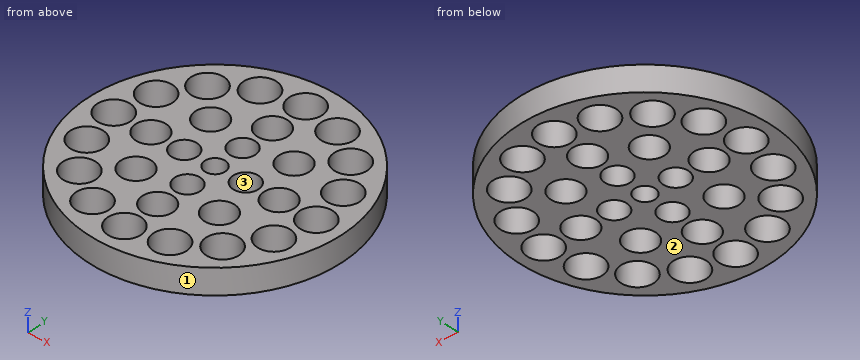
from build123d import *

# Parameters (mm, degrees)
F0_R     = 25
F0_R_2   = 3.25
F0_R_3   = 3
F0_R_4   = 2.5
F0_R_5   = 2
F1_DEPTH = 5


with BuildPart() as f1:
    # F0 (on Top) → F1 (new body)
    with BuildSketch(Plane.XY):
        Circle(F0_R)
        with Locations((-13.965359, -13.965359)):
            Circle(F0_R_2, mode=Mode.SUBTRACT)
        with Locations((-7.557998, -18.246621)):
            Circle(F0_R_2, mode=Mode.SUBTRACT)
        with Locations((-18.246621, -7.557998)):
            Circle(F0_R_2, mode=Mode.SUBTRACT)
        with Locations((-8.131728, -8.131728)):
            Circle(F0_R_3, mode=Mode.SUBTRACT)
        with Locations((0, -19.75)):
            Circle(F0_R_2, mode=Mode.SUBTRACT)
        with Locations((7.557998, -18.246621)):
            Circle(F0_R_2, mode=Mode.SUBTRACT)
        with Locations((13.965359, -13.965359)):
            Circle(F0_R_2, mode=Mode.SUBTRACT)
        with Locations((0, -12.5)):
            Circle(F0_R_3, mode=Mode.SUBTRACT)
        with Locations((8.131728, -8.131728)):
            Circle(F0_R_3, mode=Mode.SUBTRACT)
        with Locations((0, -6)):
            Circle(F0_R_4, mode=Mode.SUBTRACT)
        with Locations((18.246621, -7.557998)):
            Circle(F0_R_2, mode=Mode.SUBTRACT)
        with Locations((-19.75, 0)):
            Circle(F0_R_2, mode=Mode.SUBTRACT)
        with Locations((-18.246621, 7.557998)):
            Circle(F0_R_2, mode=Mode.SUBTRACT)
        with Locations((-12.5, 0)):
            Circle(F0_R_3, mode=Mode.SUBTRACT)
        with Locations((-6, 0)):
            Circle(F0_R_4, mode=Mode.SUBTRACT)
        with Locations((-8.131728, 8.131728)):
            Circle(F0_R_3, mode=Mode.SUBTRACT)
        with Locations((-13.965359, 13.965359)):
            Circle(F0_R_2, mode=Mode.SUBTRACT)
        with Locations((-7.557998, 18.246621)):
            Circle(F0_R_2, mode=Mode.SUBTRACT)
        Circle(F0_R_5, mode=Mode.SUBTRACT)
        with Locations((6, 0)):
            Circle(F0_R_4, mode=Mode.SUBTRACT)
        with Locations((0, 6)):
            Circle(F0_R_4, mode=Mode.SUBTRACT)
        with Locations((8.131728, 8.131728)):
            Circle(F0_R_3, mode=Mode.SUBTRACT)
        with Locations((12.5, 0)):
            Circle(F0_R_3, mode=Mode.SUBTRACT)
        with Locations((19.75, 0)):
            Circle(F0_R_2, mode=Mode.SUBTRACT)
        with Locations((18.246621, 7.557998)):
            Circle(F0_R_2, mode=Mode.SUBTRACT)
        with Locations((0, 12.5)):
            Circle(F0_R_3, mode=Mode.SUBTRACT)
        with Locations((7.557998, 18.246621)):
            Circle(F0_R_2, mode=Mode.SUBTRACT)
        with Locations((0, 19.75)):
            Circle(F0_R_2, mode=Mode.SUBTRACT)
        with Locations((13.965359, 13.965359)):
            Circle(F0_R_2, mode=Mode.SUBTRACT)
    extrude(amount=F1_DEPTH)


solid = f1.part
Read the model definition and answer for the solid it produces. Units are mm, in the model's axes. Face numbers are marked on the shaded views. Round coordinates to 2 decimals unless told otherwise and drop trailing zeros. Loops run counter-clockwise (first coordinate to the right, second up) from the corner with the lowest first, then second, coordinate; pieces in that order, holes last.
Q1. Section A-A on y = 0 is taken. Give the number of separate pieces and of enclosed holes in the cut face, and give its area (3 significant figures).
Q2. Consider probe 1 along Y at (x, z) = (6.5, 4.35); probe 2 along X at (y, z) = (13.5, 3.55); probe 3 along Y at (x, z) = (-5.5, 1). Determine where each line is inside the solid, lowest interval first.
Q3. Section B-B on x = 13.5 is taken. Write down the section's boundary in (y, z).
Q4. Each of these flat-tipped pins is pushed along its axis until it touches: pin 1 (3 mm diameter, centred on x = 4.5, z = 3, fed in from +Y); pin 2 (3 mm diameter, centred on x = 0, y = 0, fed in from -Z); pin 3 (1 mm diameter, centred on y = 15, z = 1.5, fed in from +X). Where does it stop, or does it pass through?
Q5. Determine the mould class of the marked faces 1, 2 and 3 for opening direction Y: released by +Y, released by -Y, zero draft, split by the parting line, or undercut.
Q6. Section C-C on y = 6 is taken. Write down the section's boundary in (x, z).
Output:
1. separate pieces: 8
1. enclosed holes: 0
1. area: 55.0 mm2
2. probe 1: y = -24.14 to -21.32, -15.17 to -10.65, -5.61 to -2.45, 2.45 to 5.61, 10.65 to 15.17, 21.32 to 24.14
2. probe 2: x = -21.04 to -17.18, -10.75 to -2.83, 2.83 to 10.75, 17.18 to 21.04
2. probe 3: y = -24.39 to -20.76, -15.73 to -9.57, -6.69 to -2.45, 2.45 to 6.69, 9.57 to 15.73, 20.76 to 24.39
3. outline: (-21.04, 0) - (-17.18, 0) - (-17.18, 5) - (-21.04, 5) - close; (-10.75, 0) - (-2.83, 0) - (-2.83, 5) - (-10.75, 5) - close; (2.83, 0) - (10.75, 0) - (10.75, 5) - (2.83, 5) - close; (17.18, 0) - (21.04, 0) - (21.04, 5) - (17.18, 5) - close
4. pin 1: stops at y = 24.82
4. pin 2: passes through
4. pin 3: stops at x = 20.37
5. face 1: split by the parting line
5. face 2: zero draft
5. face 3: undercut
6. outline: (-24.27, 0) - (-21.1, 0) - (-21.1, 5) - (-24.27, 5) - close; (-15.39, 0) - (-10.24, 0) - (-10.24, 5) - (-15.39, 5) - close; (-6.02, 0) - (-2.5, 0) - (-2.5, 5) - (-6.02, 5) - close; (2.5, 0) - (6.02, 0) - (6.02, 5) - (2.5, 5) - close; (10.24, 0) - (15.39, 0) - (15.39, 5) - (10.24, 5) - close; (21.1, 0) - (24.27, 0) - (24.27, 5) - (21.1, 5) - close
